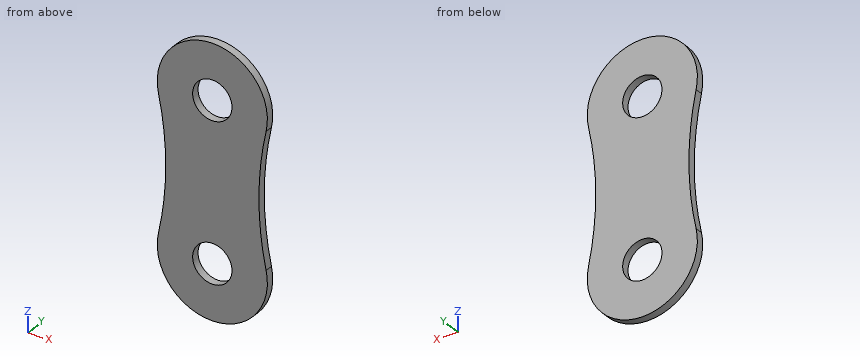
from build123d import *

# Parameters (mm, degrees)
F0_R     = 2.5
F1_DEPTH = 1
F2_R     = 2.5
F3_DEPTH = 1


with BuildPart() as f1:
    # F0 (on Front) → F1 (new body)
    with BuildSketch(Plane.XZ):
        with BuildLine():
            ThreePointArc((-6.8397, 18.511913), (-5.9237, 10.000689), (-6.8397, 1.489464))
            ThreePointArc((-6.8397, 1.489464), (0, -7), (6.8397, 1.489464))
            ThreePointArc((6.8397, 1.489464), (5.9237, 10.000689), (6.8397, 18.511913))
            ThreePointArc((6.8397, 18.511913), (0, 27.001378), (-6.8397, 18.511913))
        make_face()
        with Locations((0, 20.001378)):
            Circle(F0_R, mode=Mode.SUBTRACT)
    extrude(amount=F1_DEPTH)

    # F2 (on face) → F3 (cut)
    with BuildSketch(Plane.XZ.offset(1)):
        Circle(F2_R)
    extrude(amount=-F3_DEPTH, mode=Mode.SUBTRACT)


solid = f1.part
Could you check a few things on this model? Use its own coordinates, in mm. Give positions to 0.01 mm unless a question says otherwise; leave off trailing zeros. Order: outer loops, then holes, each group sorted by start corner. A loop starts at its lowest first (then second) coordinate and runs counter-clockwise, first axis right, second up. Notation, with made-up numbers: M 54,46.5 L 68,46.5 A25 ccw 68,68.5 Z; hole C -29.5,1 d11. An arc over 180 degrees is marked long. One line per question, with ' | ' between items.
1. I want a section at A-A (x = 0). List the corners of the cut face in (y, z) for me.
Results:
outline: M -1,-7 L 0,-7 L 0,-2.5 L -1,-2.5 Z; M -1,2.5 L 0,2.5 L 0,17.5 L -1,17.5 Z; M -1,22.5 L 0,22.5 L 0,27 L -1,27 Z
2. I want a section at C-C (y = -0.4). List the corners of the cut face in (x, z) for me, and give its area (3 significant figures).
Results:
outline: M -6.84,1.49 A7 ccw long 6.84,1.49 A40 cw 6.84,18.51 A7 ccw long -6.84,18.51 A40 cw Z; hole C 0,0 d5; hole C 0,20 d5 | area: 368 mm²
3. If I drill on line 1 (Z direction, x = 1, y = -0.8); line 2 (X direction, y = -0.8, z = 2); line 3 (X direction, y = -0.4, z = 9.5), over which ranges is the centre line in solid material (lowest first)?
Results:
line 1: -6.93 to -2.29, 2.29 to 17.71, 22.29 to 26.93 | line 2: -6.73 to -1.5, 1.5 to 6.73 | line 3: -5.93 to 5.93
4. I want a section at B-B (z = 0). List the corners of the cut face in (x, y) for me.
Results:
outline: M -7,-1 L -2.5,-1 L -2.5,0 L -7,0 Z; M 2.5,-1 L 7,-1 L 7,0 L 2.5,0 Z
5. I want a section at D-D (x = 1.5). List the corners of the cut face in (y, z) for me.
Results:
outline: M -1,-6.84 L 0,-6.84 L 0,-2 L -1,-2 Z; M -1,2 L 0,2 L 0,18 L -1,18 Z; M -1,22 L 0,22 L 0,26.84 L -1,26.84 Z
